The model under review builds one solid part; all positions refer to its coordinate system, in mm. A direction names the side the tool comes from. Give positions to 0.01 mm unless a question says otherwise; leave off trailing zeros. Order: outer loops, then holes, each group sorted by start corner. A loop starts at its lowest first (then second) coordinate and runs counter-clockwise, first axis right, second up.
```python
from build123d import *

# Parameters (mm, degrees)
EXTRUDE_1_DEPTH = 3.5
SKETCH_2_R      = 2.5
EXTRUDE_2_DEPTH = 34
CHAMFER_1_SIZE  = 0.445


with BuildPart() as part:
    # Эскиз1 → Бобышка-Вытянуть1 (new body)
    with BuildSketch(Plane.XY):
        Polygon((0.728296009, 4.561021624), (-3.585812589, 2.911233657), (-4.314108598, -1.649787967), (-0.728296009, -4.561021624), (3.585812589, -2.911233657), (4.314108598, 1.649787967), align=None)
    extrude(amount=EXTRUDE_1_DEPTH)

    # Эскиз2 → Бобышка-Вытянуть2 (add)
    with BuildSketch(Plane.XY.offset(3.5)):
        Circle(SKETCH_2_R)
    extrude(amount=EXTRUDE_2_DEPTH)

    # Фаска1
    chamfer_1_edges = [part.edges().sort_by_distance(p)[0] for p in [
        (-2.5, 0, 37.5),
    ]]
    chamfer(chamfer_1_edges, length=CHAMFER_1_SIZE)

    # Эскиз4 → Вырез-Повернуть1 (revolve, cut)
    with BuildSketch(Plane(origin=(0, 0, 0), x_dir=(1, 0, 0), z_dir=(0, 1, 0))):
        Polygon((3.5, 0), (7.5, 0), (7.5, -2.309401077), align=None)
    revolve(axis=Axis((0, 0, 0), (0, 0, 1)), mode=Mode.SUBTRACT)


solid = part.part
```
1. Take a section at B-B (z = 3). Write out the cut boundary in (x, y).
2. To check wall thickness, follow line 1 (Z direction, x = 0, y = -3.25); line 2 (Z direction, x = 0.5, y = -2); line 3 (Y direction, x = 0, z = 34.5). State the ranges of each line that lie inside material, in increasing order.
3. Take a section at D-D (z = 31.5). Write out the cut boundary in (x, y), and give its area (3 significant figures).
4. Insertion check: pin 1 (4.5 mm diameter, centred on x = -1.5, y = -1.5, fed in from +Z); pin 2 (3 mm diameter, centred on y = 1.5, z = 18.5, fed in from -X); pin 3 (1 mm diameter, centred on x = 3.5, z = 29, fed in from -Y); pin 4 (3 mm diameter, centred on x = 0.5, z = 28, fed in from +Y). Each pin has a flat end and moves straight along its axis. Give the tip position at first contact, or say it passes through.
5. Take a section at C-C (x = 0). Write out the cut boundary in (y, z) (1 decimal), and give its area (3 significant figures).
6. For faces 1 (the cylindrical face through (-0.54, -2.44, 20.04)), 2 (the flat face through (1.399, -3.748, 1.872)), list the 3-axis set-ups (+Z, -Z, +X, -X, +Y, -Y) from which the entire face can be reached by the end or side of a thin tool; tool diameter is ignored.
7. Take a section at A-A (y = 0). Write out the cut boundary in (x, z) (3 decimals), and give its area (3 significant figures).
Answer:
1. outline: (-4.31, -1.65) - (-0.73, -4.56) - (3.59, -2.91) - (4.31, 1.65) - (0.73, 4.56) - (-3.59, 2.91) - close
2. line 1: z = 0 to 3.5
2. line 2: z = 0 to 37.49
2. line 3: y = -2.5 to 2.5
3. outline: circle Ø5 at (0, 0)
3. area: 19.6 mm2
4. pin 1: stops at z = 37.5
4. pin 2: stops at x = -2.5
4. pin 3: passes through
4. pin 4: stops at y = 2.5
5. outline: (-4.3, 0.5) - (-3.5, 0) - (3.5, 0) - (4.3, 0.5) - (4.3, 3.5) - (2.5, 3.5) - (2.5, 37.1) - (2.1, 37.5) - (-2.1, 37.5) - (-2.5, 37.1) - (-2.5, 3.5) - (-4.3, 3.5) - close
5. area: 199 mm2
6. face 1: +Z
6. face 2: +Z, -Z, +X, -Y
7. outline: (-4.051, 0.318) - (-3.5, 0) - (3.5, 0) - (4.051, 0.318) - (4.051, 3.5) - (2.5, 3.5) - (2.5, 37.055) - (2.055, 37.5) - (-2.055, 37.5) - (-2.5, 37.055) - (-2.5, 3.5) - (-4.051, 3.5) - close
7. area: 198 mm2
